Input: part model. Units: mm. Frame: model coordinates. Coordinates: 2 decimals unless noted, no trailing zeros. Loops run counter-clockwise (first coordinate to the right, second up) from the corner with the lowest first, then second, coordinate; pieces in that order, holes last.
(1) Section B-B, the plane z = -34. Return loops of the section in (x, y), then the cut area to 3 significant figures.
(2) Line query: L1, parallel to Z at x = 2.5, y = 1.5; L2, parallel to X at y = 4.25, z = -33; L3, parallel to Z at x = -56, y = 1.75. Output: solid intervals per line, ascending.
(3) Contact query for flat-ended pins moving along their axis: P1, Ø8, axis at x = -82, z = -21.5, coming from the -Y side; P2, Ø3, axis at y = 3, z = -77.5, coming from the -X side; P3, Ø3, axis at x = -48, y = 4, coming from the +Z side; P4, Ø3, axis at x = -78, y = 4, coming from the -Z side. Output: stop coordinate, or through.
(4) Section A-A, the plane x = -111. Return loops of the section in (y, z).
Autodesk Inventor part; units mm, degrees
ref_plane "YZ Plane" through (0, 0, 0) normal (1, 0, 0) x (0, 1, 0)
ref_plane "XZ Plane" through (0, 0, 0) normal (0, 1, 0) x (-1, 0, 0)
ref_plane "XY Plane" through (0, 0, 0) normal (0, 0, 1) x (1, 0, 0)
sketch "Sketch1" plane through (0, 0, 0) normal (0, 1, 0) x (-1, 0, 0)
  line L0 (0, 0) -> (127, 0)
  line L1 (127, 0) -> (127, -166.624)
  line L2 (127, -166.624) -> (0, -166.624)
  line L3 (0, -166.624) -> (0, 0)
  dimension "BoxHeight" = 127
  dimension "d1" = 166.624
sketch "Sketch2" plane through (0, 0, 0) normal (0, 1, 0) x (-1, 0, 0)
  line L0 (0, 0) -> (-8.89, 0)
  line L1 (-8.89, 0) -> (-8.89, -23.8034)
  line L2 (-8.89, -23.8034) -> (0, -23.8034)
  line L3 (0, -23.8034) -> (0, 0)
  line L4 (0, -166.624) -> (0, 0)
  line L5 (0, 0) -> (127, 0)
  line L6 (0, -47.6069) -> (-8.89, -47.6069)
  line L7 (-8.89, -47.6069) -> (-8.89, -71.4103)
  line L8 (-8.89, -71.4103) -> (0, -71.4103)
  line L9 (0, -71.4103) -> (0, -47.6069)
  line L10 (0, -95.2137) -> (-8.89, -95.2137)
  line L11 (-8.89, -95.2137) -> (-8.89, -119.0171)
  line L12 (-8.89, -119.0171) -> (0, -119.0171)
  line L13 (0, -119.0171) -> (0, -95.2137)
  line L14 (63.5, 0) -> (63.5, -115.824) construction
  line L15 (127, -23.8034) -> (127, 0)
  line L16 (127, -166.624) -> (127, 0)
  line L17 (127, -71.4103) -> (127, -47.6069)
  line L18 (127, -119.0171) -> (127, -95.2137)
  line L19 (28.2222, -166.624) -> (14.1111, -166.624)
  line L20 (14.1111, -166.624) -> (14.1111, -175.514)
  line L21 (14.1111, -175.514) -> (28.2222, -175.514)
  line L22 (28.2222, -175.514) -> (28.2222, -166.624)
  line L23 (127, -166.624) -> (0, -166.624)
  line L24 (56.4444, -166.624) -> (42.3333, -166.624)
  line L25 (42.3333, -166.624) -> (42.3333, -175.514)
  line L26 (42.3333, -175.514) -> (56.4444, -175.514)
  line L27 (56.4444, -175.514) -> (56.4444, -166.624)
  line L28 (84.6667, -166.624) -> (70.5556, -166.624)
  line L29 (70.5556, -166.624) -> (70.5556, -175.514)
  line L30 (70.5556, -175.514) -> (84.6667, -175.514)
  line L31 (84.6667, -175.514) -> (84.6667, -166.624)
  line L32 (112.8889, -166.624) -> (98.7778, -166.624)
  line L33 (98.7778, -166.624) -> (98.7778, -175.514)
  line L34 (98.7778, -175.514) -> (112.8889, -175.514)
  line L35 (112.8889, -175.514) -> (112.8889, -166.624)
  line L36 (127, -83.312) -> (0, -83.312) construction
  line L37 (63.5, -166.624) -> (63.5, -50.8) construction
  line L38 (28.2222, 0) -> (14.1111, 0)
  line L39 (14.1111, 0) -> (14.1111, 8.89)
  line L40 (14.1111, 8.89) -> (28.2222, 8.89)
  line L41 (28.2222, 8.89) -> (28.2222, 0)
  line L42 (127, 0) -> (0, 0)
  line L43 (56.4444, 0) -> (42.3333, 0)
  line L44 (42.3333, 0) -> (42.3333, 8.89)
  line L45 (42.3333, 8.89) -> (56.4444, 8.89)
  line L46 (56.4444, 8.89) -> (56.4444, 0)
  line L47 (84.6667, 0) -> (70.5556, 0)
  line L48 (70.5556, 0) -> (70.5556, 8.89)
  line L49 (84.6667, 8.89) -> (84.6667, 0)
  line L50 (70.5556, 8.89) -> (84.6667, 8.89)
  line L51 (112.8889, 0) -> (98.7778, 0)
  line L52 (98.7778, 0) -> (98.7778, 8.89)
  line L53 (112.8889, 8.89) -> (112.8889, 0)
  line L54 (98.7778, 8.89) -> (112.8889, 8.89)
  line L55 (0, -142.8206) -> (-8.89, -142.8206)
  line L56 (-8.89, -142.8206) -> (-8.89, -159.3669)
  line L57 (-8.89, -159.3669) -> (0, -159.3669)
  line L58 (0, -159.3669) -> (0, -142.8206)
  line L59 (127, -166.624) -> (127, 0)
  line L60 (127, 0) -> (135.89, 0)
  line L61 (135.89, 0) -> (135.89, -23.8034)
  line L62 (135.89, -23.8034) -> (127, -23.8034)
  line L63 (127, -23.8034) -> (127, 0)
  line L64 (127, -166.624) -> (127, 0)
  line L65 (127, -47.6069) -> (135.89, -47.6069)
  line L66 (135.89, -47.6069) -> (135.89, -71.4103)
  line L67 (135.89, -71.4103) -> (127, -71.4103)
  line L68 (127, -71.4103) -> (127, -47.6069)
  line L69 (127, -95.2137) -> (135.89, -95.2137)
  line L70 (135.89, -95.2137) -> (135.89, -119.0171)
  line L71 (135.89, -119.0171) -> (127, -119.0171)
  line L72 (127, -119.0171) -> (127, -95.2137)
  line L73 (135.89, -142.8206) -> (135.89, -159.3669)
  line L74 (127, -142.8206) -> (135.89, -142.8206)
  line L75 (127, -159.3669) -> (127, -142.8206)
  line L76 (135.89, -159.3669) -> (127, -159.3669)
  line L77 (14.1111, -175.514) -> (0, -175.514)
  line L78 (0, -175.514) -> (0, -159.3669)
  line L79 (0, -159.3669) -> (14.1111, -159.3669)
  line L80 (14.1111, -159.3669) -> (14.1111, -175.514)
  line L81 (28.2222, -175.514) -> (42.3333, -175.514)
  line L82 (42.3333, -175.514) -> (42.3333, -166.624)
  line L83 (42.3333, -166.624) -> (28.2222, -166.624)
  line L84 (28.2222, -166.624) -> (28.2222, -175.514)
  line L85 (56.4444, -175.514) -> (70.5556, -175.514)
  line L86 (70.5556, -175.514) -> (70.5556, -166.624)
  line L87 (70.5556, -166.624) -> (56.4444, -166.624)
  line L88 (56.4444, -166.624) -> (56.4444, -175.514)
  line L89 (84.6667, -175.514) -> (98.7778, -175.514)
  line L90 (98.7778, -175.514) -> (98.7778, -166.624)
  line L91 (98.7778, -166.624) -> (84.6667, -166.624)
  line L92 (84.6667, -166.624) -> (84.6667, -175.514)
  line L93 (112.8889, -175.514) -> (127, -175.514)
  line L94 (127, -175.514) -> (127, -159.3669)
  line L95 (127, -159.3669) -> (112.8889, -159.3669)
  line L96 (112.8889, -159.3669) -> (112.8889, -175.514)
  line L97 (112.8889, 0) -> (127, 0)
  line L98 (127, 0) -> (127, 8.89)
  line L99 (127, 8.89) -> (112.8889, 8.89)
  line L100 (112.8889, 8.89) -> (112.8889, 0)
  line L101 (98.7778, 8.89) -> (84.6667, 8.89)
  line L102 (84.6667, 8.89) -> (84.6667, 0)
  line L103 (84.6667, 0) -> (98.7778, 0)
  line L104 (98.7778, 0) -> (98.7778, 8.89)
  line L105 (70.5556, 8.89) -> (56.4444, 8.89)
  line L106 (56.4444, 8.89) -> (56.4444, 0)
  line L107 (56.4444, 0) -> (70.5556, 0)
  line L108 (70.5556, 0) -> (70.5556, 8.89)
  line L109 (42.3333, 8.89) -> (28.2222, 8.89)
  line L110 (28.2222, 8.89) -> (28.2222, 0)
  line L111 (28.2222, 0) -> (42.3333, 0)
  line L112 (42.3333, 0) -> (42.3333, 8.89)
  line L113 (14.1111, 8.89) -> (0, 8.89)
  line L114 (0, 8.89) -> (0, 0)
  line L115 (0, 0) -> (14.1111, 0)
  line L116 (14.1111, 0) -> (14.1111, 8.89)
  line L117 (0, 0) -> (-8.89, 0)
  line L118 (-8.89, 0) -> (-8.89, 8.89)
  line L119 (-8.89, 8.89) -> (0, 8.89)
  line L120 (0, 8.89) -> (0, 0)
  line L121 (0, -159.3669) -> (-8.89, -159.3669)
  line L122 (-8.89, -159.3669) -> (-8.89, -168.2569)
  line L123 (-8.89, -168.2569) -> (0, -168.2569)
  line L124 (0, -168.2569) -> (0, -159.3669)
  line L125 (127, -159.3669) -> (135.89, -159.3669)
  line L126 (135.89, -159.3669) -> (135.89, -168.2569)
  line L127 (135.89, -168.2569) -> (127, -168.2569)
  line L128 (127, -168.2569) -> (127, -159.3669)
  line L129 (127, 0) -> (135.89, 0)
  line L130 (135.89, 0) -> (135.89, 8.89)
  line L131 (135.89, 8.89) -> (127, 8.89)
  line L132 (127, 8.89) -> (127, 0)
  line L133 (127, -168.2569) -> (135.89, -168.2569)
  line L134 (135.89, -168.2569) -> (135.89, -175.514)
  line L135 (135.89, -175.514) -> (127, -175.514)
  line L136 (127, -175.514) -> (127, -168.2569)
  line L137 (0, -168.2569) -> (-8.89, -168.2569)
  line L138 (-8.89, -168.2569) -> (-8.89, -175.514)
  line L139 (-8.89, -175.514) -> (0, -175.514)
  line L140 (0, -175.514) -> (0, -168.2569)
  dimension "d2" = 8.89
  dimension "d3" = 23.8034
  dimension "d5" = 8.89
  dimension "d6" = 23.8034
  dimension "d7" = 23.8034
  dimension "d8" = 8.89
  dimension "d9" = 23.8034
  dimension "d10" = 23.8034
  dimension "d11" = 14.1111
  dimension "d12" = 127
  dimension "d13" = 14.1111
  dimension "d14" = 8.89
  dimension "d15" = 8.89
  dimension "d16" = 14.1111
  dimension "d17" = 8.89
  dimension "d18" = 14.1111
  dimension "d22" = 8.89
  dimension "d23" = 14.1111
  dimension "d27" = 14.1111
  dimension "d28" = 14.1111
  dimension "d29" = 14.1111
  dimension "d34" = 8.89
  dimension "d35" = 16.5463
  dimension "d40" = 23.8034
  dimension "d41" = 8.89
  dimension "d42" = 8.89
  dimension "d43" = 8.89
  dimension "d44" = 8.89
  dimension "d45" = 8.89
  dimension "d46" = 8.89
  dimension "d47" = 8.89
  dimension "d48" = 8.89
extrude "Connections" add sketch "Sketch2" along normal blind 6.35 contours L3 L2 L1 L0 | L114 L113 L39 L5 | L0 L118 L119 L114 | L4 L8 L7 L6 | L41 L109 L44 L5 | L4 L12 L11 L10 | L46 L105 L48 L5 | L4 L57 L56 L55 | L49 L101 L52 L5 | L79 L80 L23 L4 | L4 L78 L123 L122 L57 | L23 L20 L77 L78 | L53 L99 L98 L5 | L78 L139 L138 L123 | L60 L61 L62 L15 | L98 L131 L130 L60 | L23 L25 L81 L22 | L65 L66 L67 L16 | L23 L29 L85 L27 | L69 L70 L71 L16 | L23 L33 L89 L31 | L74 L73 L76 L16 | L96 L95 L16 L23 | L23 L94 L93 L35 | L76 L126 L127 L94 L16 | L94 L127 L134 L135
extrude "Base Extrusion" add sketch "Sketch1" along normal blind 6.35
sketch "Sketch3" plane through (0, 6.35, 0) normal (0, 1, 0) x (1, 0, 0)
  line L0 (-6.2788, 64.0613) -> (-6.2788, 44.7093) construction
  line L1 (-6.2788, 44.7093) -> (-46.5625, 44.7093) construction
  line L2 (-46.5625, 44.7093) -> (-46.5625, 64.0613) construction
  line L3 (-46.5625, 64.0613) -> (-6.2788, 64.0613) construction
  point P0 (0, 0)
sketch "Sketch4" plane through (0, 6.35, 0) normal (0, 1, 0) x (1, 0, 0)
  point P0 (0, 0)
sketch "Sketch5" plane through (0, 6.35, 0) normal (0, 1, 0) x (1, 0, 0)
  line L0 (-127, 119.0171) -> (-135.89, 119.0171)
  line L1 (-135.89, 119.0171) -> (-135.89, 95.2137)
  line L2 (-135.89, 95.2137) -> (-127, 95.2137)
  line L3 (-127, 95.2137) -> (-127, 71.4103)
  line L4 (-127, 71.4103) -> (-135.89, 71.4103)
  line L5 (-135.89, 71.4103) -> (-135.89, 47.6069)
  line L6 (-135.89, 47.6069) -> (-127, 47.6069)
  line L7 (-127, 47.6069) -> (-127, 23.8034)
  line L8 (-127, 23.8034) -> (-135.89, 23.8034)
  line L9 (-135.89, 23.8034) -> (-135.89, -8.89)
  line L10 (-135.89, -8.89) -> (-112.8889, -8.89)
  line L11 (-112.8889, -8.89) -> (-112.8889, 0)
  line L12 (-112.8889, 0) -> (-98.7778, 0)
  line L13 (-98.7778, 0) -> (-98.7778, -8.89)
  line L14 (-98.7778, -8.89) -> (-84.6667, -8.89)
  line L15 (-84.6667, -8.89) -> (-84.6667, 0)
  line L16 (-84.6667, 0) -> (-70.5556, 0)
  line L17 (-70.5556, 0) -> (-70.5556, -8.89)
  line L18 (-70.5556, -8.89) -> (-56.4444, -8.89)
  line L19 (-56.4444, -8.89) -> (-56.4444, 0)
  line L20 (-56.4444, 0) -> (-42.3333, 0)
  line L21 (-42.3333, 0) -> (-42.3333, -8.89)
  line L22 (-42.3333, -8.89) -> (-28.2222, -8.89)
  line L23 (-28.2222, -8.89) -> (-28.2222, 0)
  line L24 (-28.2222, 0) -> (-14.1111, 0)
  line L25 (-14.1111, 0) -> (-14.1111, -8.89)
  line L26 (-14.1111, -8.89) -> (8.89, -8.89)
  line L27 (8.89, -8.89) -> (8.89, 23.8034)
  line L28 (8.89, 23.8034) -> (0, 23.8034)
  line L29 (0, 23.8034) -> (0, 47.6069)
  line L30 (0, 47.6069) -> (8.89, 47.6069)
  line L31 (8.89, 47.6069) -> (8.89, 71.4103)
  line L32 (8.89, 71.4103) -> (0, 71.4103)
  line L33 (0, 71.4103) -> (0, 95.2137)
  line L34 (0, 95.2137) -> (8.89, 95.2137)
  line L35 (8.89, 95.2137) -> (8.89, 119.0171)
  line L36 (8.89, 119.0171) -> (0, 119.0171)
  line L37 (0, 119.0171) -> (0, 142.8206)
  line L38 (0, 142.8206) -> (8.89, 142.8206)
  line L39 (8.89, 142.8206) -> (8.89, 175.514)
  line L40 (8.89, 175.514) -> (-14.1111, 175.514)
  line L41 (-14.1111, 175.514) -> (-14.1111, 166.624)
  line L42 (-14.1111, 166.624) -> (-28.2222, 166.624)
  line L43 (-28.2222, 166.624) -> (-28.2222, 175.514)
  line L44 (-28.2222, 175.514) -> (-42.3333, 175.514)
  line L45 (-42.3333, 175.514) -> (-42.3333, 166.624)
  line L46 (-42.3333, 166.624) -> (-56.4444, 166.624)
  line L47 (-56.4444, 166.624) -> (-56.4444, 175.514)
  line L48 (-56.4444, 175.514) -> (-70.5556, 175.514)
  line L49 (-70.5556, 175.514) -> (-70.5556, 166.624)
  line L50 (-70.5556, 166.624) -> (-84.6667, 166.624)
  line L51 (-84.6667, 166.624) -> (-84.6667, 175.514)
  line L52 (-84.6667, 175.514) -> (-98.7778, 175.514)
  line L53 (-98.7778, 175.514) -> (-98.7778, 166.624)
  line L54 (-98.7778, 166.624) -> (-112.8889, 166.624)
  line L55 (-112.8889, 166.624) -> (-112.8889, 175.514)
  line L56 (-112.8889, 175.514) -> (-135.89, 175.514)
  line L57 (-135.89, 175.514) -> (-135.89, 142.8206)
  line L58 (-135.89, 142.8206) -> (-127, 142.8206)
  line L59 (-127, 142.8206) -> (-127, 119.0171)
  point P0 (0, 0)
equation "\"d1\" = BaseWidth"
equation "\"d2\" = WallConA"
equation "\"d3\" = WallConB"
equation "\"d5\" = d2"
equation "\"d6\" = WallConSpace"
equation "\"d7\" = d4"
equation "\"d8\" = d2"
equation "\"d9\" = d6"
equation "\"d10\" = d4"
equation "\"d11\" = -0.8 * d13 + 0.2 * d12"
equation "\"d13\" = 0.111111 * d12"
equation "\"d14\" = WallConA"
equation "\"d15\" = d14"
equation "\"d16\" = d13"
equation "\"d17\" = d15"
equation "\"d18\" = d20"
equation "\"d22\" = d17"
equation "\"d23\" = d25"
equation "\"d27\" = d11"
equation "\"d28\" = d27"
equation "\"d29\" = d11"
equation "\"d34\" = d36"
equation "\"d35\" = d37"
equation "\"d40\" = d7"
equation "\"d41\" = d5"
equation "\"d42\" = d5"
equation "\"d43\" = d41"
equation "\"d44\" = d42"
equation "\"d45\" = d41"
equation "\"d46\" = d42"
equation "\"d47\" = d41"
equation "\"d48\" = d42"
equation "\"d4\" = WallConSpace"
equation "\"d20\" = 0.111111 * d21"
equation "\"d25\" = 0.111111 * d26"
equation "\"d36\" = d38"
equation "\"d37\" = d39"
properties part number "WallToWall"
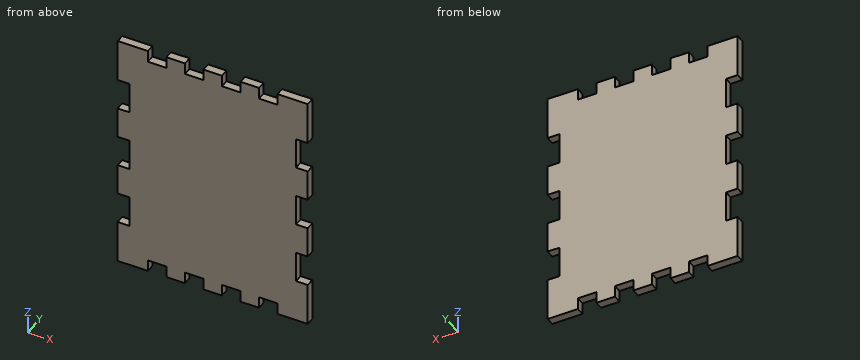
Report:
1. outline: (-127, 0) - (0, 0) - (0, 6.35) - (-127, 6.35) - close
1. area: 806 mm2
2. L1: z = -175.51 to -142.82, -119.02 to -95.21, -71.41 to -47.61, -23.8 to 8.89
2. L2: x = -127 to 0
2. L3: z = -166.62 to 0
3. P1: stops at y = 0
3. P2: stops at x = -127
3. P3: stops at z = 0
3. P4: stops at z = -166.62
4. outline: (0, -166.62) - (6.35, -166.62) - (6.35, 0) - (0, 0) - close
